Verification items for the finished model (mm, model axes). Face numbers are marked on the shaded views. A direction names the side the tool comes from. Give positions to 0.01 mm unless a question says otherwise; leave off trailing zeros. Write each loop counter-clockwise with the first axis right and the second up, starting at its lowest first coordinate (ties: lowest second). Pieces come first, ordered by that corner, then holes. Notation, with made-up numbers: M -18,-3 L 11,-3 A15 ccw 11,3 Z; hole C 68,31 d6. An arc over 180 degrees is marked long. Write item = value, one per line.
from build123d import *

# Parameters (mm, degrees)
ESBO_O1_W                = 6
ESBO_O1_H                = 6
ESBO_O1_H_2              = 1
ESBO_O1_H_3              = 1.5
RESSALTO_EXTRUS_O1_DEPTH = 4
ESBO_O2_W                = 30
ESBO_O2_H                = 39
ESBO_O2_W_2              = 3.5
ESBO_O2_H_2              = 23
RESSALTO_EXTRUS_O2_DEPTH = 1.5
RESSALTO_EXTRUS_O2_TAPER = 27
ESBO_O3_W                = 1
ESBO_O3_H                = 1
RESSALTO_EXTRUS_O3_DEPTH = 6.5
ESBO_O4_W                = 16
ESBO_O4_H                = 20
ESBO_O4_W_2              = 10
ESBO_O4_H_2              = 15
RESSALTO_EXTRUS_O4_DEPTH = 1.6
RESSALTO_EXTRUS_O4_DRAFT = 25


with BuildPart() as part:
    # Esboço1 → Ressalto-extrusão1 (new body)
    with BuildSketch(Plane.XY):
        Polygon((13.5, 25), (13.5, 19), (13.5, 0), (13.5, -4), (13.5, -11), (6, -11), (6, -12.5), (15, -12.5), (15, 0), (15, 26.5), (0, 26.5), (-15, 26.5), (-15, 0), (-15, -12.5), (-6, -12.5), (-6, -11), (-13.5, -11), (-13.5, -4), (-13.5, 0), (-13.5, 19), (-13.5, 25), (0, 25), align=None)
        Polygon((-10, 0), (-7.5, 0), (-7.5, 19), (-7.5, 24), (-12.5, 24), (-12.5, 19), (-10, 19), align=None)
        Polygon((7.5, 19), (7.5, 0), (10, 0), (10, 19), (12.5, 19), (12.5, 24), (7.5, 24), align=None)
        Polygon((7.5, 0), (0, 0), (-7.5, 0), (-10, 0), (-10, -4), (-6, -4), (0, -4), (6, -4), (10, -4), (10, 0), align=None)
        Polygon((-6, -4), (-10, -4), (-12.5, -4), (-12.5, -10), (-6, -10), align=None)
        Polygon((-12.5, -10), (-12.5, -4), (-13.5, -4), (-13.5, -11), (-6, -11), (-6, -10), align=None)
        Polygon((12.5, -4), (10, -4), (6, -4), (6, -10), (12.5, -10), align=None)
        Polygon((13.5, -4), (12.5, -4), (12.5, -10), (6, -10), (6, -11), (13.5, -11), align=None)
        with Locations((-3, -7)):
            Rectangle(ESBO_O1_W, ESBO_O1_H)
        with Locations((3, -7)):
            Rectangle(ESBO_O1_W, ESBO_O1_H)
        with Locations((3, -10.5)):
            Rectangle(ESBO_O1_W, ESBO_O1_H_2)
        with Locations((-3, -10.5)):
            Rectangle(ESBO_O1_W, ESBO_O1_H_2)
        with Locations((-3, -11.75)):
            Rectangle(ESBO_O1_W, ESBO_O1_H_3)
        with Locations((3, -11.75)):
            Rectangle(ESBO_O1_W, ESBO_O1_H_3)
    extrude(amount=RESSALTO_EXTRUS_O1_DEPTH)

    # Esboço2 → Ressalto-extrusão2 (add)
    with BuildSketch(Plane.XY.offset(4)):
        with Locations((0, 7)):
            Rectangle(ESBO_O2_W, ESBO_O2_H)
        with Locations((11.75, 7.5)):
            Rectangle(ESBO_O2_W_2, ESBO_O2_H_2, mode=Mode.SUBTRACT)
        with Locations((-11.75, 7.5)):
            Rectangle(ESBO_O2_W_2, ESBO_O2_H_2, mode=Mode.SUBTRACT)
    extrude(amount=RESSALTO_EXTRUS_O2_DEPTH, taper=RESSALTO_EXTRUS_O2_TAPER)

    # Esboço3 → Ressalto-extrusão3 (add)
    with BuildSketch(Plane.XY.offset(5.5)):
        Polygon((7, 16), (7, 0), (7, -1), (7, -2), (8, -2), (8, 18), (-8, 18), (-8, -2), (-7, -2), (-7, -1), (-7, 0), (-7, 16), (-7, 17), (-6, 17), (6, 17), (7, 17), align=None)
        with Locations((-6.5, -1.5)):
            Rectangle(ESBO_O3_W, ESBO_O3_H)
        with Locations((-6.5, -0.5)):
            Rectangle(ESBO_O3_W, ESBO_O3_H)
        with Locations((-6.5, 16.5)):
            Rectangle(ESBO_O3_W, ESBO_O3_H)
        with Locations((6.5, 16.5)):
            Rectangle(ESBO_O3_W, ESBO_O3_H)
        with Locations((6.5, -0.5)):
            Rectangle(ESBO_O3_W, ESBO_O3_H)
        with Locations((6.5, -1.5)):
            Rectangle(ESBO_O3_W, ESBO_O3_H)
    extrude(amount=RESSALTO_EXTRUS_O3_DEPTH)


with BuildPart() as ressalto_extrus_o4_tool:
    # Esboço4 → Ressalto-extrusão4 (with draft: the straight prism first)
    with BuildSketch(Plane.XY.offset(12)):
        with Locations((0, 8)):
            Rectangle(ESBO_O4_W, ESBO_O4_H)
        with Locations((0, 7.5)):
            Rectangle(ESBO_O4_W_2, ESBO_O4_H_2, mode=Mode.SUBTRACT)
    extrude(amount=RESSALTO_EXTRUS_O4_DEPTH)
    # Ressalto-extrusão4: the draft: its side faces are tilted about the plane it starts from
    ressalto_extrus_o4_sides = [ressalto_extrus_o4_tool.faces().sort_by_distance(p)[0] for p in [
        (-8, 8, 12.8),
        (0, -2, 12.8),
        (8, 8, 12.8),
        (0, 18, 12.8),
        (0, 15, 12.8),
        (5, 7.5, 12.8),
        (0, 0, 12.8),
        (-5, 7.5, 12.8),
    ]]
    draft(ressalto_extrus_o4_sides, Plane.XY.offset(12), RESSALTO_EXTRUS_O4_DRAFT)


with BuildPart() as part_1:
    add(part.part)

    # Ressalto-extrusão4: add ressalto_extrus_o4_tool
    add(ressalto_extrus_o4_tool.part)


solid = part_1.part
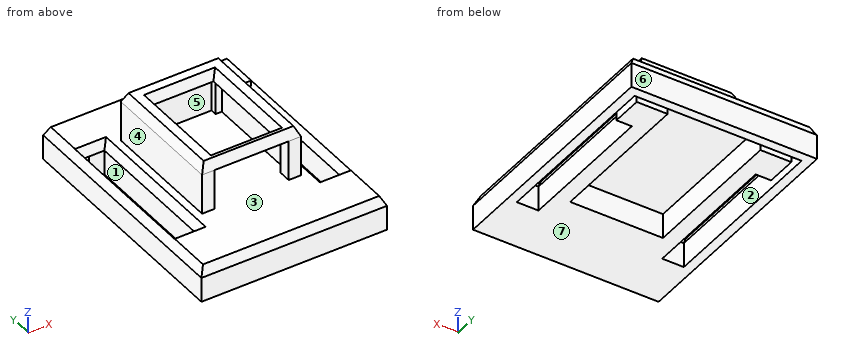
1) Material ranges on probe 1 along X at (y, z) = (16, 3.75); probe 2 along X at (y, z) = (-0.5, 2.25); probe 3 along X at (y, z) = (2.5, 9.25), recorded low to high. Write a range as from..to.
From the geometry:
probe_1 = -15..-13.5, -10..-7.5, 7.5..10, 13.5..15
probe_2 = -15..-13.5, -10..10, 13.5..15
probe_3 = -8..-7, 7..8
2) Cross-section at B-B on y = 16.5. Count the separate pieces of the cut face and the enclosed holes in it, plus the area to 3 significant figures.
From the geometry:
separate_pieces = 3
enclosed_holes = 1
area = 113 mm^2
3) Tool access check on the marked faces 1, 2, 3 and 4. Record the directions out of +Z, -Z, +X, -X, +Y, -Y that give a thin tool (end or side, any length) a straight path to the whole face; none if there is none.
From the geometry:
face_1 = +Z, -Z
face_2 = -Z
face_3 = none
face_4 = +Z, -X, +Y, -Y
4) Cross-section at D-D on z = 6.25. Record the boundary of the cut face in (x, y).
From the geometry:
outline = M -8,-2 L -6,-2 L -6,0 L -7,0 L -7,16 L -6,16 L -6,17 L 6,17 L 6,16 L 7,16 L 7,0 L 6,0 L 6,-2 L 8,-2 L 8,18 L -8,18 Z
5) Draft check along Z on the marked faces 5, 6 and 7. Enter one of: +Z half, -Z half, draft (parallel to the pull), parting line (faces both ways), or undercut.
From the geometry:
face_5 = undercut
face_6 = draft
face_7 = -Z half
6) Cross-section at A-A on z = 1. Record the boundary of the cut face in (x, y).
From the geometry:
outline = M -15,-12.5 L 15,-12.5 L 15,26.5 L -15,26.5 Z; hole M -13.5,-4 L -10,-4 L -10,19 L -12.5,19 L -12.5,24 L -7.5,24 L -7.5,0 L 7.5,0 L 7.5,24 L 12.5,24 L 12.5,19 L 10,19 L 10,-4 L 13.5,-4 L 13.5,25 L -13.5,25 Z
7) Depth check by flat-ended pin: P1, Ø2, axis at x = -2, z = 10.5, coming from the -Y side; P2, Ø1.1, axis at x = 6.5, z = 9, coming from the +Y side; P3, Ø0.8, axis at y = 16.5, z = 8, coming from the -X side; P4, Ø5, axis at x = -3.5, y = -2, coming from the +Z side. Enter the tip coordinate at first touch or a pass-through.
From the geometry:
P1 = 17
P2 = 18
P3 = -8
P4 = 13.6
